The listing builds one solid part. Answer for the finished solid, in the listing's coordinates (mm). Give positions to 0.01 mm unless a question says otherwise; leave off trailing zeros. Write each loop counter-clockwise with the first axis right and the second up, starting at its lowest first coordinate (ties: lowest second). Pieces come first, ordered by that corner, then holes. Notation, with made-up numbers: (71, 5.25) - (100, 5.25) arc R14 ccw to (100, 30.25) - close; hole circle Ø7 at (44.5, 21.5). An arc over 180 degrees is marked (long way). Use a Markdown table: item, result. Add a question column.
from build123d import *

# Parameters (mm, degrees)
SKETCH1_W           = 300
SKETCH1_H           = 12
BOSS_EXTRUDE1_DEPTH = 8
CHAMFER1_SIZE       = 1
SKETCH2_R           = 2.95
CUT_EXTRUDE1_DEPTH  = 5.05
SKETCH3_R           = 1.825
CUT_EXTRUDE2_DEPTH  = 151.332963784
LPATTERN2_COUNT     = 12
LPATTERN2_PITCH     = 24.65


with BuildPart() as part:
    # Sketch1 → Boss-Extrude1 (new body)
    with BuildSketch(Plane(origin=(0, 0, 0), x_dir=(1, 0, 0), z_dir=(0, 1, 0))):
        Rectangle(SKETCH1_W, SKETCH1_H)
    extrude(amount=BOSS_EXTRUDE1_DEPTH)

    # Chamfer1
    chamfer1_edges = [part.edges().sort_by_distance(p)[0] for p in [
        (0, 8, -6),
        (0, 0, -6),
        (0, 0, 6),
        (0, 8, 6),
    ]]
    chamfer(chamfer1_edges, length=CHAMFER1_SIZE)

    # Sketch2 → Cut-Extrude1 (cut)
    with BuildSketch(Plane(origin=(0, 0, 0), x_dir=(1, 0, 0), z_dir=(0, 1, 0))):
        with Locations(Location((137.05, 0, 0), (0, 0, 270))):
            Circle(SKETCH2_R)
    cut_extrude1 = extrude(amount=CUT_EXTRUDE1_DEPTH, mode=Mode.SUBTRACT)

    # Sketch3 → Cut-Extrude2 (cut, through all)
    with BuildSketch(Plane(origin=(0, 0, 0), x_dir=(1, 0, 0), z_dir=(0, 1, 0))):
        with Locations(Location((137.05, 0, 0), (0, 0, 270))):
            Circle(SKETCH3_R)
    cut_extrude2 = extrude(amount=CUT_EXTRUDE2_DEPTH, mode=Mode.SUBTRACT)

    # LPattern2: Cut-Extrude1, Cut-Extrude2 ×12
    with Locations(*[(-i * LPATTERN2_PITCH, 0, 0) for i in range(1, LPATTERN2_COUNT)]):
        add(cut_extrude1, mode=Mode.SUBTRACT)
        add(cut_extrude2, mode=Mode.SUBTRACT)


solid = part.part
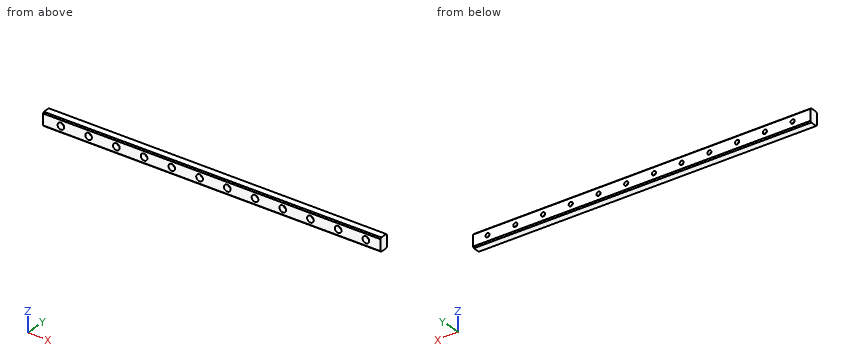
1. Given P1, Ø2, axis at x = -35.5, z = 0, coming from the -Y side; P2, Ø4.5, axis at x = -10.85, z = 0, coming from the -Y side, each flat-ended and moving along its own axis, determine where each tip first touches the part or whether it passes through.
2. The part is cut by section A-A (y = 2.75). Count the separate pieces of the cut face and the enclosed holes in it, and give its area (3 significant figures).
3. The part is cut by section B-B (x = 50.5). Give the vertices of the cut face in (y, z).
4. Consider L1, parallel to Z at x = 137.05, y = 2.5; L2, parallel to Y at x = -60.5, z = 2; L3, parallel to Z at x = 112.4, y = 5.7 (3 decimals). Determine where each line is inside the solid, lowest interval first. Write a range as [from, to].
Check values:
| question | item | result |
|---|---|---|
| 1 | P1 | passes through |
| 1 | P2 | stops at y = 5.05 |
| 2 | separate pieces | 1 |
| 2 | enclosed holes | 12 |
| 2 | area | 3,270 mm2 |
| 3 | outline | (0, -5) - (1, -6) - (7, -6) - (8, -5) - (8, 5) - (7, 6) - (1, 6) - (0, 5) - close |
| 4 | L1 | z = [-6, -2.95], [2.95, 6] |
| 4 | L2 | y = [5.05, 8] |
| 4 | L3 | z = [-6, -1.825], [1.825, 6] |
